from build123d import *

# Parameters (mm, degrees)
PRIMARY_START           = -25.4
SKETCH2_W               = 66
SKETCH2_H               = 60
SKETCH2_R               = 1.5875
SKETCH2_H_2             = 92.4
PRIMARY_EXTRUSION_DEPTH = 62.5
CUT_EXTRUDE2_START      = -25.4
SKETCH3_R               = 3.175
CUT_EXTRUDE2_DEPTH      = 25.4
CUT_EXTRUDE3_START      = -87.9
SKETCH2_4_R             = 1.5875
CUT_EXTRUDE3_DEPTH      = 6.35
CHAMFER1_SIZE           = 1.5875
CUT_EXTRUDE4_DEPTH      = 6.35
CUT_EXTRUDE5_OUTLINE_R  = 8
CUT_EXTRUDE5_DEPTH      = 152.4


# Read off the part's stored shape, not the designer's step: Cut-Extrude5
with BuildPart() as part:
    # Sketch2 → Primary Extrusion (new body)
    # profile 1 of 10: a face of its own
    with BuildSketch(Plane.XY.offset(PRIMARY_START)):
        with Locations((112.625, 30)):
            Rectangle(SKETCH2_W, SKETCH2_H)
        with BuildLine():
            ThreePointArc((88.925, 7), (85.625, 3.7), (82.325, 7))
            ThreePointArc((82.325, 7), (85.625, 10.3), (88.925, 7))
        make_face(mode=Mode.SUBTRACT)
        with BuildLine():
            ThreePointArc((95.325, 7), (98.625, 10.3), (101.925, 7))
            ThreePointArc((101.925, 7), (98.625, 3.7), (95.325, 7))
        make_face(mode=Mode.SUBTRACT)
        with Locations((113.875, 23.675)):
            Circle(SKETCH2_R, mode=Mode.SUBTRACT)
        with Locations((139.275, 23.675)):
            Circle(SKETCH2_R, mode=Mode.SUBTRACT)
        with Locations((113.875, 36.325)):
            Circle(SKETCH2_R, mode=Mode.SUBTRACT)
        with Locations((139.275, 36.325)):
            Circle(SKETCH2_R, mode=Mode.SUBTRACT)
        with BuildLine():
            ThreePointArc((88.925, 53), (85.625, 49.7), (82.325, 53))
            ThreePointArc((82.325, 53), (85.625, 56.3), (88.925, 53))
        make_face(mode=Mode.SUBTRACT)
        with BuildLine():
            ThreePointArc((101.925, 53), (98.625, 49.7), (95.325, 53))
            ThreePointArc((95.325, 53), (98.625, 56.3), (101.925, 53))
        make_face(mode=Mode.SUBTRACT)
    # profile 2 of 10: a face of its own
    with BuildSketch(Plane.XY.offset(PRIMARY_START)):
        with BuildLine():
            ThreePointArc((82.325, 53), (85.625, 49.7), (88.925, 53))
            ThreePointArc((88.925, 53), (85.625, 56.3), (82.325, 53))
        make_face()
    # profile 3 of 10: a face of its own
    with BuildSketch(Plane.XY.offset(PRIMARY_START)):
        with BuildLine():
            ThreePointArc((95.325, 53), (98.625, 49.7), (101.925, 53))
            ThreePointArc((101.925, 53), (98.625, 56.3), (95.325, 53))
        make_face()
    # profile 4 of 10: a face of its own
    with BuildSketch(Plane.XY.offset(PRIMARY_START)):
        with Locations((113.875, 36.325)):
            Circle(SKETCH2_R)
    # profile 5 of 10: a face of its own
    with BuildSketch(Plane.XY.offset(PRIMARY_START)):
        with Locations((113.875, 23.675)):
            Circle(SKETCH2_R)
    # profile 6 of 10: a face of its own
    with BuildSketch(Plane.XY.offset(PRIMARY_START)):
        with Locations((139.275, 36.325)):
            Circle(SKETCH2_R)
    # profile 7 of 10: a face of its own
    with BuildSketch(Plane.XY.offset(PRIMARY_START)):
        with Locations((139.275, 23.675)):
            Circle(SKETCH2_R)
    # profile 8 of 10: a face of its own
    with BuildSketch(Plane.XY.offset(PRIMARY_START)):
        with BuildLine():
            ThreePointArc((82.325, 7), (85.625, 3.7), (88.925, 7))
            ThreePointArc((88.925, 7), (85.625, 10.3), (82.325, 7))
        make_face()
    # profile 9 of 10: a face of its own
    with BuildSketch(Plane.XY.offset(PRIMARY_START)):
        with BuildLine():
            ThreePointArc((101.925, 7), (98.625, 10.3), (95.325, 7))
            ThreePointArc((95.325, 7), (98.625, 3.7), (101.925, 7))
        make_face()
    # profile 10 of 10: a face of its own
    with BuildSketch(Plane.XY.offset(PRIMARY_START)):
        with Locations((112.625, 106.2)):
            Rectangle(SKETCH2_W, SKETCH2_H_2)
    extrude(amount=-PRIMARY_EXTRUSION_DEPTH)

    # Sketch3 → Cut-Extrude2 (cut)
    with BuildSketch(Plane.XY.offset(CUT_EXTRUDE2_START)):
        with Locations((-135.5, 47.3)):
            Circle(SKETCH3_R)
        with Locations((-135.5, 12.7)):
            Circle(SKETCH3_R)
        with Locations((93.595, 47.3)):
            Circle(SKETCH3_R)
        with Locations((131.655, 47.3)):
            Circle(SKETCH3_R)
        with Locations((131.655, 12.7)):
            Circle(SKETCH3_R)
        with Locations((93.595, 12.7)):
            Circle(SKETCH3_R)
    extrude(amount=-CUT_EXTRUDE2_DEPTH, mode=Mode.SUBTRACT)

    # Sketch2<4> → Cut-Extrude3 (cut)
    with BuildSketch(Plane.XY.offset(CUT_EXTRUDE3_START)):
        with BuildLine():
            ThreePointArc((95.325, 53), (98.625, 49.7), (101.925, 53))
            ThreePointArc((101.925, 53), (98.625, 56.3), (95.325, 53))
        make_face()
        with BuildLine():
            ThreePointArc((82.325, 53), (85.625, 49.7), (88.925, 53))
            ThreePointArc((88.925, 53), (85.625, 56.3), (82.325, 53))
        make_face()
        with BuildLine():
            ThreePointArc((101.925, 7), (98.625, 10.3), (95.325, 7))
            ThreePointArc((95.325, 7), (98.625, 3.7), (101.925, 7))
        make_face()
        with BuildLine():
            ThreePointArc((82.325, 7), (85.625, 3.7), (88.925, 7))
            ThreePointArc((88.925, 7), (85.625, 10.3), (82.325, 7))
        make_face()
        with Locations((139.275, 36.325)):
            Circle(SKETCH2_4_R)
        with Locations((113.875, 36.325)):
            Circle(SKETCH2_4_R)
        with Locations((113.875, 23.675)):
            Circle(SKETCH2_4_R)
        with Locations((139.275, 23.675)):
            Circle(SKETCH2_4_R)
    extrude(amount=CUT_EXTRUDE3_DEPTH, mode=Mode.SUBTRACT)

    # Chamfer1
    chamfer1_edges = [part.edges().sort_by_distance(p)[0] for p in [
        (112.625, 0, -25.4),
        (79.625, 76.2, -25.4),
        (145.625, 76.2, -25.4),
    ]]
    chamfer(chamfer1_edges, length=CHAMFER1_SIZE)

    # Sketch4 → Cut-Extrude4 (cut)
    with BuildSketch(Plane(origin=(0, 0, 0), x_dir=(1, 0, 0), z_dir=(0, 1, 0))):
        with BuildLine():
            ThreePointArc((131.310028843, 75.335028843), (134.060028843, 78.085028843), (136.810028843, 75.335028843))
            ThreePointArc((136.810028843, 75.335028843), (134.060028843, 72.585028843), (131.310028843, 75.335028843))
        make_face()
        with BuildLine():
            ThreePointArc((117.875, 80.9), (120.625, 83.65), (123.375, 80.9))
            ThreePointArc((123.375, 80.9), (120.625, 78.15), (117.875, 80.9))
        make_face()
        with BuildLine():
            ThreePointArc((104.439971157, 75.335028843), (107.189971157, 78.085028843), (109.939971157, 75.335028843))
            ThreePointArc((109.939971157, 75.335028843), (107.189971157, 72.585028843), (104.439971157, 75.335028843))
        make_face()
        with BuildLine():
            ThreePointArc((104.439971157, 48.464971157), (107.189971157, 51.214971157), (109.939971157, 48.464971157))
            ThreePointArc((109.939971157, 48.464971157), (107.189971157, 45.714971157), (104.439971157, 48.464971157))
        make_face()
        with BuildLine():
            ThreePointArc((123.375, 42.9), (120.625, 40.15), (117.875, 42.9))
            ThreePointArc((117.875, 42.9), (120.625, 45.65), (123.375, 42.9))
        make_face()
        with BuildLine():
            ThreePointArc((136.810028843, 48.464971157), (134.060028843, 45.714971157), (131.310028843, 48.464971157))
            ThreePointArc((131.310028843, 48.464971157), (134.060028843, 51.214971157), (136.810028843, 48.464971157))
        make_face()
    extrude(amount=CUT_EXTRUDE4_DEPTH, mode=Mode.SUBTRACT)

    # Cut-Extrude5 outline → Cut-Extrude5 (cut)
    with BuildSketch(Plane(origin=(0, 0, 0), x_dir=(1, 0, 0), z_dir=(0, 1, 0))):
        with Locations((120.625, 61.9)):
            Circle(CUT_EXTRUDE5_OUTLINE_R)
    extrude(amount=CUT_EXTRUDE5_DEPTH, mode=Mode.SUBTRACT)


solid = part.part
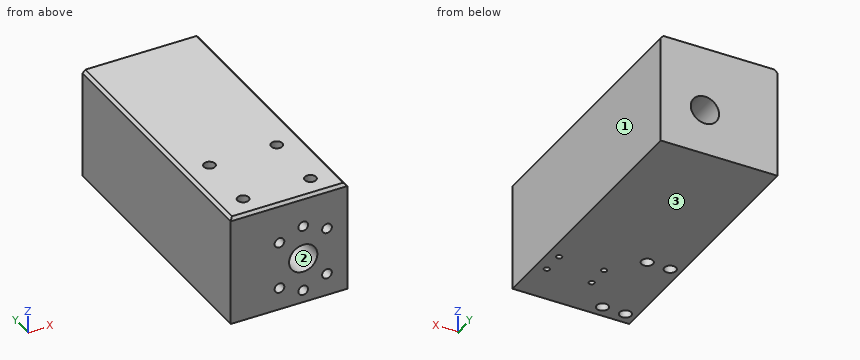
Geometry check sheet. Reference: the model listing, model coordinates, mm. Face numbers are marked on the shaded views. Give positions to 0.01 mm unless a question says otherwise; leave off trailing zeros. Order: outer loops, then holes, each group sorted by start corner. A loop starts at its lowest first (then second) coordinate and runs counter-clockwise, first axis right, second up. Notation, with made-up numbers: (-1, 60) - (21, 60) arc R25 ccw to (21, 84) - close; hole circle Ø2 at (42.5, 31.5). An arc over 180 degrees is marked (long way). Use one line per item in the form item = value.
1) Depth check by flat-ended pin: pin 1 Ø3 at (x, y) = (113.875, 36.325) entering from -Z; pin 2 Ø5.5 at (x, y) = (131.655, 47.3) entering from +Z. Enter the tip coordinate at first touch or a pass-through.
Working result:
pin_1 = -81.55
pin_2 = -50.8
2) Sectioned sample at D-D (y = 47.3). Record the boundary of the cut face in (x, z) (1 decimal), and give its area (3 significant figures).
Working result:
outline = (79.6, -87.9) - (145.6, -87.9) - (145.6, -27) - (144, -25.4) - (134.8, -25.4) - (134.8, -50.8) - (128.5, -50.8) - (128.5, -25.4) - (96.8, -25.4) - (96.8, -50.8) - (90.4, -50.8) - (90.4, -25.4) - (81.2, -25.4) - (79.6, -27) - close; hole circle Ø16 at (120.6, -61.9)
area = 3,600 mm^2
3) Sectioned sample at B-B (z = -42.9). Record the boundary of the cut face in (x, y) (3 decimals), and give its area (3 significant figures).
Working result:
outline = (79.625, 0) - (117.875, 0) - (117.875, 6.35) - (123.375, 6.35) - (123.375, 0) - (145.625, 0) - (145.625, 152.4) - (79.625, 152.4) - close; hole circle Ø6.35 at (93.595, 12.7); hole circle Ø6.35 at (93.595, 47.3); hole circle Ø6.35 at (131.655, 12.7); hole circle Ø6.35 at (131.655, 47.3)
area = 9,900 mm^2
4) Material ranges on probe 1 along X at (y, z) = (45, -46.5) (3 decimals); probe 2 along Y at (x, z) = (94.5, -31); probe 3 along Z at (x, y) = (125, 74), recorded low to high. Write a range as from..to.
Working result:
probe_1 = 79.625..91.406, 95.784..129.466, 133.844..145.625
probe_2 = 0..9.66, 15.74..44.26, 50.34..152.4
probe_3 = -87.9..-68.6, -55.2..-25.4
5) Draft check along Z on the marked faces 1, 2 and 3. Enter one of: released by +Z, released by -Z, zero draft, split by the parting line, or undercut.
Working result:
face_1 = zero draft
face_2 = undercut
face_3 = released by -Z
6) Sectioned sample at A-A (y = 122.5). Record the boundary of the cut face in (x, z) (1 decimal), and give its area (3 significant figures).
Working result:
outline = (79.6, -87.9) - (145.6, -87.9) - (145.6, -27) - (144, -25.4) - (81.2, -25.4) - (79.6, -27) - close; hole circle Ø16 at (120.6, -61.9)
area = 3,920 mm^2
7) Sectioned sample at C-C (z = -61.9). Record the boundary of the cut face in (x, y) (3 decimals), and give its area (3 significant figures).
Working result:
outline = (79.625, 0) - (112.625, 0) - (112.625, 152.4) - (79.625, 152.4) - close; (128.625, 0) - (145.625, 0) - (145.625, 152.4) - (128.625, 152.4) - close
area = 7,620 mm^2
